Job drawing, mm, ordinate dimensions from the low corner. One solid piece. Give positions to 0.01 mm unless a question says otherwise; leave off trailing zeros. Order: outer loops, then holes, each group sorted by start corner. A loop starts at its lowest first (then second) coordinate and runs counter-clockwise, first axis right, second up. Notation, with made-up numbers: (-2, 52.25) -> (56, 52.25) arc R27 cw to (56, 89.25) -> close; hole circle Ø7 at (-2.75, 30.25). An arc over 180 degrees is marked (long way). Write item = value, one per line. Start each with the question number.
(1) Probe line 1 along X through (y, z) = (4, 16); line 2 along Z through (x, y) = (33, 3.5); line 3 along X through (y, z) = (2.75, 46.5). List the from-to ranges inside material, lowest first. Write a range as from..to.
(2) Saw through at B-B, the plane z = 37.5. List the corners of the cut face in (x, y).
(3) Two-plate mould, pull along Y, no slides. Class the marked faces 1 and 2: pulls with the +Y half, pulls with the -Y half, needs draft (parallel to the pull), parting line crosses it, or undercut.
(4) Saw through at A-A, the plane z = 26.67. List the corners of the cut face in (x, y).
(5) Saw through at C-C, the plane x = 24.5. List the corners of the cut face in (y, z).
(6) Saw through at D-D, the plane y = 1.25. State how many separate pieces and enclosed holes the cut face has, then the cut area to 3 significant figures.
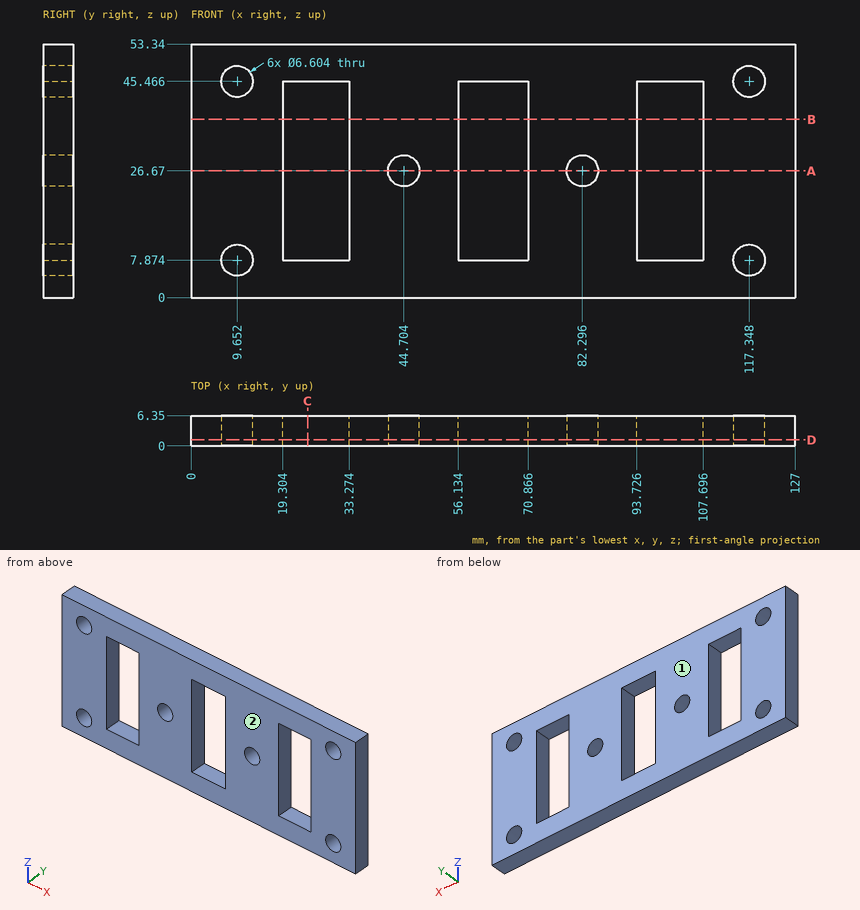
Results list:
q1.line_1 = 0..19.3, 33.27..56.13, 70.87..93.73, 107.7..127
q1.line_2 = 0..7.87, 45.47..53.34
q1.line_3 = 0..6.52, 12.79..114.21, 120.48..127
q2.outline = (0, 0) -> (19.3, 0) -> (19.3, 6.35) -> (0, 6.35) -> close; (33.27, 0) -> (56.13, 0) -> (56.13, 6.35) -> (33.27, 6.35) -> close; (70.87, 0) -> (93.73, 0) -> (93.73, 6.35) -> (70.87, 6.35) -> close; (107.7, 0) -> (127, 0) -> (127, 6.35) -> (107.7, 6.35) -> close
q3.face_1 = pulls with the +Y half
q3.face_2 = pulls with the -Y half
q4.outline = (0, 0) -> (19.3, 0) -> (19.3, 6.35) -> (0, 6.35) -> close; (33.27, 0) -> (41.4, 0) -> (41.4, 6.35) -> (33.27, 6.35) -> close; (48.01, 0) -> (56.13, 0) -> (56.13, 6.35) -> (48.01, 6.35) -> close; (70.87, 0) -> (78.99, 0) -> (78.99, 6.35) -> (70.87, 6.35) -> close; (85.6, 0) -> (93.73, 0) -> (93.73, 6.35) -> (85.6, 6.35) -> close; (107.7, 0) -> (127, 0) -> (127, 6.35) -> (107.7, 6.35) -> close
q5.outline = (0, 0) -> (6.35, 0) -> (6.35, 7.87) -> (0, 7.87) -> close; (0, 45.47) -> (6.35, 45.47) -> (6.35, 53.34) -> (0, 53.34) -> close
q6.separate_pieces = 1
q6.enclosed_holes = 9
q6.area = 4,960 mm^2
